For this review, use the dimensioned drawing (mm, ordinates from the lowest corner) and the shaded views. Coordinates: 2 decimals unless noted, no trailing zeros. Write each loop counter-clockwise with the first axis right and the second up, starting at its lowest first coordinate (ties: lowest second). Pieces come first, ordered by that corner, then holes. Notation, with made-up numbers: (-1.75, 29.5) - (11.25, 29.5) arc R30 cw to (11.25, 67.5) - close; hole circle Ø1 at (19, 44). An arc over 180 degrees is marked (long way). Use one line per item in the form item = value. Start each with the question number.
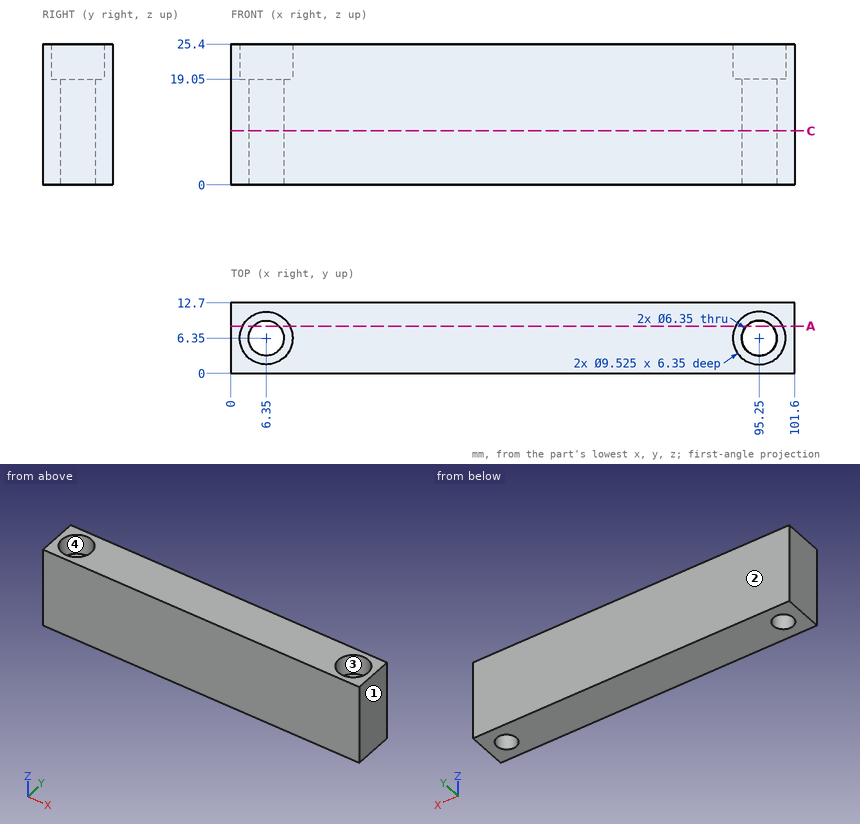
1. The part is to be moulded in two halves that separate along Y. For the marked faces 1, 2, 3 and 4, say which applies: released by +Y, released by -Y, zero draft, split by the parting line, or undercut.
2. For P1, Ø4, axis at x = 6.35, y = 6.35, coming from the -Z side; P2, Ø3, axis at x = 97, y = 7.5, coming from the +Z side, all flat-tipped, find the tip position at first contact; note any pin that passes through.
3. For L1, parallel to X at y = 6, z = 5.25; L2, parallel to X at y = 6.35, z = 24; L3, parallel to Y at x = 95.25, z = 8 (3 decimals), list the stretches that pass through material, from the lowest coordinate up.
4. Take a section at C-C (z = 9.75). State the section outline as (x, y) points (3 decimals), plus the area to 3 significant figures.
5. Take a section at A-A (y = 8.5). State the section outline as (x, z) points.
Returned:
q1.face_1 = zero draft
q1.face_2 = released by +Y
q1.face_3 = undercut
q1.face_4 = undercut
q2.P1 = through
q2.P2 = 19.05
q3.L1 = 0 to 3.19, 9.51 to 92.09, 98.41 to 101.6
q3.L2 = 0 to 1.59, 11.11 to 90.49, 100.01 to 101.6
q3.L3 = 0 to 3.175, 9.525 to 12.7
q4.outline = (0, 0) - (101.6, 0) - (101.6, 12.7) - (0, 12.7) - close; hole circle Ø6.35 at (6.35, 6.35); hole circle Ø6.35 at (95.25, 6.35)
q4.area = 1,230 mm²
q5.outline = (0, 0) - (4.01, 0) - (4.01, 19.05) - (2.1, 19.05) - (2.1, 25.4) - (0, 25.4) - close; (8.69, 0) - (92.91, 0) - (92.91, 19.05) - (91, 19.05) - (91, 25.4) - (10.6, 25.4) - (10.6, 19.05) - (8.69, 19.05) - close; (97.59, 0) - (101.6, 0) - (101.6, 25.4) - (99.5, 25.4) - (99.5, 19.05) - (97.59, 19.05) - close
